from build123d import *

# Parameters (mm, degrees)
ESQUISSE1_W             = 160
ESQUISSE1_H             = 90
EXTRUSION1_DEPTH        = 50
CONG_1_R                = 25
CONG_2_R                = 15
COQUE1_T                = -7
ESQUISSE2_W             = 50
ESQUISSE2_H             = 15
ENL_V_MAT_EXTRU_1_DEPTH = 5
CONG_4_R                = 5
CONG_5_R                = 5
CONG_6_R                = 5
CONG_7_R                = 5
CONG_4_OF_SYM_TRIE1_R   = 5
CONG_5_OF_SYM_TRIE1_R   = 5
CONG_6_OF_SYM_TRIE1_R   = 5
CONG_7_OF_SYM_TRIE1_R   = 5
ECHELLE1_SCALE          = 1.125


with BuildPart() as part:
    # Esquisse1 → Extrusion1 (new body)
    with BuildSketch(Plane(origin=(0, 0, 0), x_dir=(1, 0, 0), z_dir=(0, 1, 0))):
        with Locations((35.341232877, 23.705753425)):
            Rectangle(ESQUISSE1_W, ESQUISSE1_H)
    extrude(amount=EXTRUSION1_DEPTH)

    # Congé1
    cong_1_edges = [part.edges().sort_by_distance(p)[0] for p in [
        (115.341232877, 50, -23.705753425),
        (-44.658767123, 50, -23.705753425),
    ]]
    fillet(cong_1_edges, radius=CONG_1_R)

    # Congé2
    cong_2_edges = [part.edges().sort_by_distance(p)[0] for p in [
        (35.341232877, 50, 21.294246575),
        (35.341232877, 50, -68.705753425),
        (115.341232877, 12.5, 21.294246575),
        (-44.658767123, 12.5, 21.294246575),
        (108.018902406, 42.67766953, 21.294246575),
        (-37.336436653, 42.67766953, 21.294246575),
        (-44.658767123, 12.5, -68.705753425),
        (115.341232877, 12.5, -68.705753425),
        (108.018902406, 42.67766953, -68.705753425),
        (-37.336436653, 42.67766953, -68.705753425),
    ]]
    fillet(cong_2_edges, radius=CONG_2_R)

    # Coque1
    coque1_openings = [part.faces().sort_by_distance(p)[0] for p in [
        (35.341232877, 0, -23.705753425),
    ]]
    offset(amount=COQUE1_T, openings=coque1_openings, kind=Kind.INTERSECTION)

    # Esquisse2 → Enlèv. mat.-Extru.1 (cut)
    with BuildSketch(Plane.XY.offset(21.294246575)):
        with Locations((35.341232877, 22.5)):
            Rectangle(ESQUISSE2_W, ESQUISSE2_H)
    enl_v_mat_extru_1 = extrude(amount=-ENL_V_MAT_EXTRU_1_DEPTH, mode=Mode.SUBTRACT)

    # Congé4
    cong_4_edges = [part.edges().sort_by_distance(p)[0] for p in [
        (35.341232877, 15, 16.294246575),
    ]]
    fillet(cong_4_edges, radius=CONG_4_R - 0.0001)  # a hair under: the kernel refuses the full size

    # Congé5
    cong_5_edges = [part.edges().sort_by_distance(p)[0] for p in [
        (35.341232877, 30, 16.294246575),
    ]]
    fillet(cong_5_edges, radius=CONG_5_R - 0.0001)  # a hair under: the kernel refuses the full size

    # Congé6
    cong_6_edges = [part.edges().sort_by_distance(p)[0] for p in [
        (10.341232877, 16.464436805, 17.75868338),
        (10.341232877, 22.5, 16.294246575),
        (10.341232877, 28.535563195, 17.75868338),
    ]]
    fillet(cong_6_edges, radius=CONG_6_R - 0.0001)  # a hair under: the kernel refuses the full size

    # Congé7
    cong_7_edges = [part.edges().sort_by_distance(p)[0] for p in [
        (60.341232877, 22.5, 16.294246575),
        (60.341232877, 16.464436805, 17.75868338),
        (60.341232877, 28.535563195, 17.75868338),
    ]]
    fillet(cong_7_edges, radius=CONG_7_R - 0.0001)  # a hair under: the kernel refuses the full size

    # Symétrie1: Enlèv. mat.-Extru.1 across plane
    add(enl_v_mat_extru_1.mirror(Plane.XY.offset(-23.705753425)), mode=Mode.SUBTRACT)

    # Congé4 of Symétrie1
    cong_4_of_sym_trie1_edges = [part.edges().sort_by_distance(p)[0] for p in [
        (35.341232877, 15, -63.705753425),
    ]]
    fillet(cong_4_of_sym_trie1_edges, radius=CONG_4_OF_SYM_TRIE1_R - 0.0001)  # a hair under: the kernel refuses the full size

    # Congé5 of Symétrie1
    cong_5_of_sym_trie1_edges = [part.edges().sort_by_distance(p)[0] for p in [
        (35.341232877, 30, -63.705753425),
    ]]
    fillet(cong_5_of_sym_trie1_edges, radius=CONG_5_OF_SYM_TRIE1_R - 0.0001)  # a hair under: the kernel refuses the full size

    # Congé6 of Symétrie1
    cong_6_of_sym_trie1_edges = [part.edges().sort_by_distance(p)[0] for p in [
        (10.341232877, 16.464436805, -65.170190229),
        (10.341232877, 22.5, -63.705753425),
        (10.341232877, 28.535563195, -65.170190229),
    ]]
    fillet(cong_6_of_sym_trie1_edges, radius=CONG_6_OF_SYM_TRIE1_R - 0.0001)  # a hair under: the kernel refuses the full size

    # Congé7 of Symétrie1
    cong_7_of_sym_trie1_edges = [part.edges().sort_by_distance(p)[0] for p in [
        (60.341232877, 22.5, -63.705753425),
        (60.341232877, 16.464436805, -65.170190229),
        (60.341232877, 28.535563195, -65.170190229),
    ]]
    fillet(cong_7_of_sym_trie1_edges, radius=CONG_7_OF_SYM_TRIE1_R - 0.0001)  # a hair under: the kernel refuses the full size


with BuildPart() as part_1:
    # Echelle1: scaled about (35.341232877, 30.549354713, -23.705753425)
    add(part.part.scale(ECHELLE1_SCALE).moved(Location((-4.41765411, -3.818669339, 2.963219178))))


solid = part_1.part
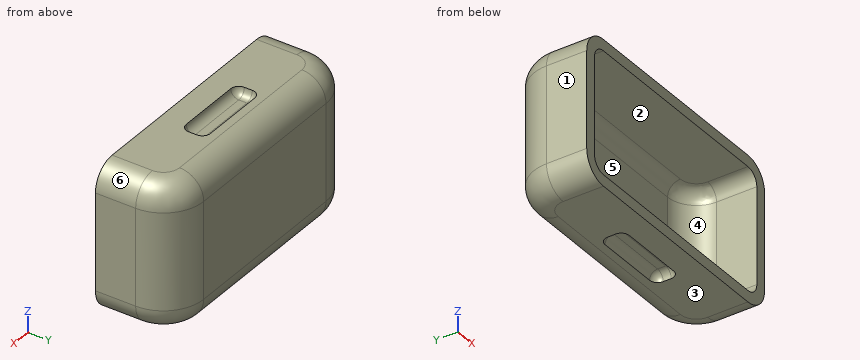
The listing builds one solid part. Answer for the finished solid, in the listing's coordinates (mm). Face numbers are marked on the shaded views. A direction names the side the tool comes from. Coordinates: 2 decimals unless noted, no trailing zeros. Write each loop counter-clockwise with the first axis right and the second up, starting at its lowest first coordinate (ties: lowest second). Pieces come first, ordered by that corner, then holes. Notation, with made-up numbers: (-11.75, 23) - (4.25, 23) arc R27 cw to (4.25, 40) - close; hole circle Ø2 at (35.25, 48.25). An arc over 180 degrees is marked (long way). Answer as CSV lines item,"result".
1. Find section C-C (z = -33.5). Give the vertices of the cut face in (x, y) (3 decimals).
Computed values:
outline,"(-54.659, -3.819) - (-46.784, -3.819) - (-46.784, 24.306) arc R20.25 cw to (-26.534, 44.556) - (97.216, 44.556) arc R20.25 cw to (117.466, 24.306) - (117.466, -3.819) - (125.341, -3.819) - (125.341, 24.306) arc R28.125 ccw to (97.216, 52.431) - (-26.534, 52.431) arc R28.125 ccw to (-54.659, 24.306) - close"
2. Find section A-A (y = 1.5). Give the vertices of the cut face in (x, z) (3 decimals), plus the area to 3 significant figures.
Computed values:
outline,"(-54.659, -57.456) arc R16.875 ccw to (-37.784, -74.331) - (108.466, -74.331) arc R16.875 ccw to (125.341, -57.456) - (125.341, 10.044) arc R16.875 ccw to (108.466, 26.919) - (-37.784, 26.919) arc R16.875 ccw to (-54.659, 10.044) - close; hole (-46.784, -57.456) arc R9 ccw to (-37.784, -66.456) - (108.466, -66.456) arc R9 ccw to (117.466, -57.456) - (117.466, 10.044) arc R9 ccw to (108.466, 19.044) - (-37.784, 19.044) arc R9 ccw to (-46.784, 10.044) - close"
area,"4,010 mm²"
3. Straight lines are drawn through the part: line 1 (X direction, y = 3.5, z = 6.5); line 2 (Z direction, x = -12, y = 6); line 3 (X direction, y = 25, z = -56.5). For each, find the intervals that lie inside material, in ascending order. Write a range as [from, to].
Computed values:
line 1,"x = [-54.66, -46.78], [117.47, 125.34]"
line 2,"z = [-74.33, -66.46], [19.04, 26.92]"
line 3,"x = [-54.65, -46.77], [117.45, 125.33]"
4. Find section B-B (x = 66). Give the vertices of the cut face in (y, z) (3 decimals).
Computed values:
outline,"(-3.819, -74.331) - (35.556, -74.331) arc R16.875 ccw to (52.431, -57.456) - (52.431, 10.044) arc R16.875 ccw to (35.556, 26.919) - (-3.819, 26.919) - (-3.819, 19.044) - (35.556, 19.044) arc R9 cw to (44.556, 10.044) - (44.556, -57.456) arc R9 cw to (35.556, -66.456) - (-3.819, -66.456) - close"
5. A tool of negligible diameter and unlimited length cuts with its end or side. For the marked faces 5 and 6, from which of +Z, -Z, +X, -X, +Y, -Y can it reach the whole face along a straight path? Write none if from no direction.
Computed values:
face 5,"-Y"
face 6,"+Z, +X, +Y, -Y"
6. Determine the mould class of the marked faces 1, 2, 3 and 4 for opening direction Z: +Z half, -Z half, draft (parallel to the pull), parting line (faces both ways), or undercut.
Computed values:
face 1,"draft"
face 2,"undercut"
face 3,"-Z half"
face 4,"undercut"
7. Given P1, Ø8, axis at x = 106.5, y = 42, coming from the -Z side; P2, Ø8, axis at x = -30.5, z = -33, coming from the -Y side; P3, Ø12, axis at x = 71, z = -37, coming from the -Y side, each flat-ended and moving along its own axis, determine where each tip first touches the part or whether it passes through.
Computed values:
P1,"stops at z = -73.65"
P2,"stops at y = 42.92"
P3,"stops at y = 44.56"
